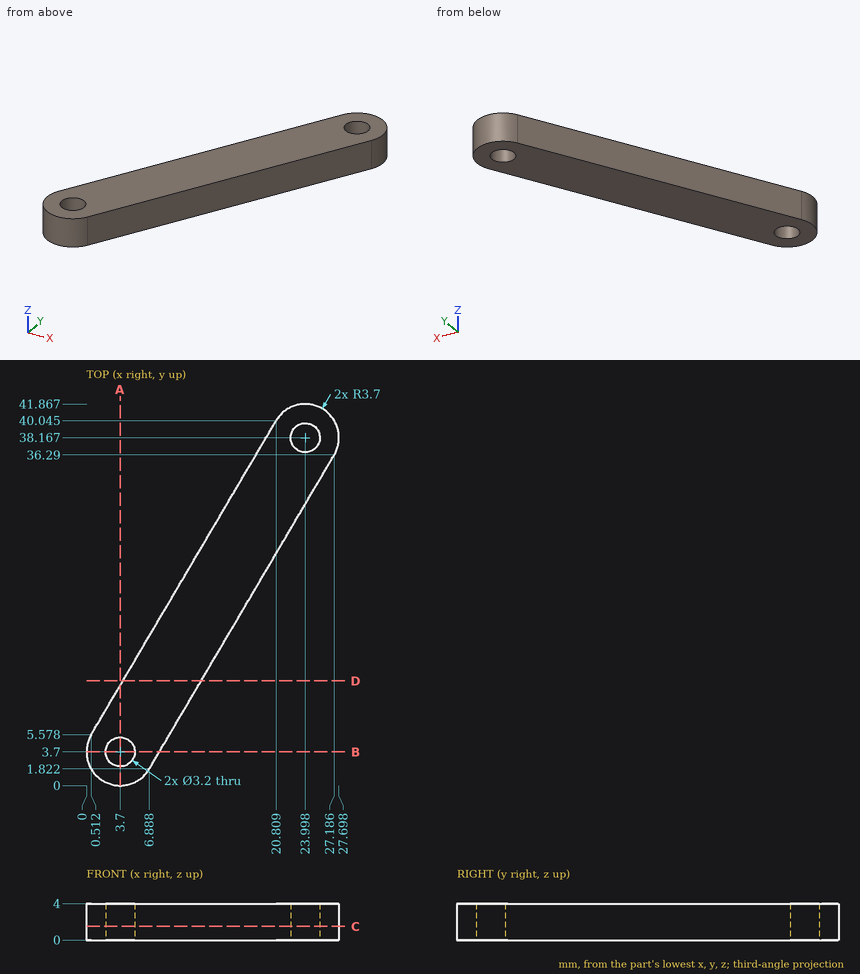
Here's the drawing with two shaded views (mm, measured from the low corner). I have some questions. Give positions to 0.01 mm unless a question says otherwise; leave off trailing zeros. Order: outer loops, then holes, each group sorted by start corner. A loop starts at its lowest first (then second) coordinate and runs counter-clockwise, first axis right, second up. Notation, with made-up numbers: M 35,57 L 82,57 A22 ccw 82,92 Z; hole C 73.25,6 d1. An arc over 180 degrees is marked long. Answer as a JSON object with one key per item and string values. Group by question number.
1) I'm going to push a flat-ended pin straight in: pin 1 Ø5 at (x, y) = (15, 35.5) entering from +Z. Where does the tip first touch, or does it pass through?
2) Suppose I cut it at D-D, the plane y = 11.5. Write out the boundary of the cut face in (x, z).
3) Suppose I cut it at C-C, the plane z = 1.5. Write out the boundary of the cut face in (x, y) (1 decimal).
4) Suppose I cut it at A-A, the plane x = 3.7. Write out the boundary of the cut face in (y, z).
5) Suppose I cut it at B-B, the plane y = 3.7. Write out the boundary of the cut face in (x, z).
6) Please list where these lines run through material, in increasing order: L1, parallel to X at y = 4, z = 3.55; L2, parallel to X at y = 3.7, z = 1.7 (1 decimal); L3, parallel to Y at x = 3.7, z = 1.6 (1 decimal). Write a range as [from, to].
Results found:
{
 "1": {"pin 1": "through"},
 "2": {"outline": "M 4,0 L 12.59,0 L 12.59,4 L 4,4 Z"},
 "3": {"outline": "M 0.5,5.6 A3.7 ccw 6.9,1.8 L 27.2,36.3 A3.7 ccw 20.8,40 Z; hole C 3.7,3.7 d3.2; hole C 24,38.2 d3.2"},
 "4": {"outline": "M 0,0 L 2.1,0 L 2.1,4 L 0,4 Z; M 5.3,0 L 10.99,0 L 10.99,4 L 5.3,4 Z"},
 "5": {"outline": "M 0,0 L 2.1,0 L 2.1,4 L 0,4 Z; M 5.3,0 L 7.99,0 L 7.99,4 L 5.3,4 Z"},
 "6": {"L1": "[0.01, 2.13], [5.27, 8.17]", "L2": "[0, 2.1], [5.3, 8]", "L3": "[0, 2.1], [5.3, 11]"}
}
